from build123d import *

# Parameters (mm, degrees)
SKETCH1_R               = 13.5
BOSS_EXTRUDE1_DEPTH     = 1.75
CUT_EXTRUDE1_DEPTH      = 20.17191957
CIRPATTERN1_COUNT       = 4
CUT_EXTRUDE2_DEPTH      = 20.17191957
CUT_EXTRUDE2_DEPTH_BACK = 20.17191957
SKETCH3_W               = 4.596194078
SKETCH3_H               = 4.596194078
CHAMFER1_SIZE           = 0.5
SKETCH4_R               = 13.5
SKETCH4_R_2             = 12.5
CUT_EXTRUDE3_DEPTH      = 1


with BuildPart() as part:
    # Sketch1 → Boss-Extrude1 (new, symmetric)
    with BuildSketch(Plane(origin=(0, 0, 0), x_dir=(0, 0, -1), z_dir=(1, 0, 0))):
        Circle(SKETCH1_R)
    extrude(amount=BOSS_EXTRUDE1_DEPTH, both=True)

    # Sketch2 → Cut-Extrude1 (cut, symmetric)
    with BuildSketch(Plane(origin=(0, 0, 0), x_dir=(0, 0, -1), z_dir=(1, 0, 0))):
        with BuildLine():
            ThreePointArc((0, 3.587478321), (-3.402339743, 6.089548883), (-5.012219469, 9.99397715))
            ThreePointArc((-5.012219469, 9.99397715), (-2.621563936, 11.159720287), (0, 11.6087119))
            ThreePointArc((0, 11.6087119), (2.621563936, 11.159720287), (5.012219469, 9.99397715))
            ThreePointArc((5.012219469, 9.99397715), (3.402339743, 6.089548883), (0, 3.587478321))
        make_face()
    cut_extrude1 = extrude(amount=CUT_EXTRUDE1_DEPTH, both=True, mode=Mode.SUBTRACT)

    # CirPattern1: Cut-Extrude1 ×4 about axis
    cirpattern1_axis = Axis((0, 0, 0), (1, 0, 0))
    for i in range(1, CIRPATTERN1_COUNT):
        add(cut_extrude1.rotate(cirpattern1_axis, i * 360 / CIRPATTERN1_COUNT), mode=Mode.SUBTRACT)

    # Sketch3 → Cut-Extrude2 (cut, two sides: drawn at the far end of the back side and taken through both)
    with BuildSketch(Plane(origin=(0, 0, 0), x_dir=(0, 0, -1), z_dir=(1, 0, 0)).offset(-CUT_EXTRUDE2_DEPTH_BACK)):
        Rectangle(SKETCH3_W, SKETCH3_H)
    extrude(amount=CUT_EXTRUDE2_DEPTH + CUT_EXTRUDE2_DEPTH_BACK, mode=Mode.SUBTRACT)

    # Chamfer1
    chamfer1_edges = [part.edges().sort_by_distance(p)[0] for p in [
        (1.75, 0, 13.5),
        (1.75, 0, 2.298097039),
        (1.75, -2.298097039, 0),
        (1.75, 0, -2.298097039),
        (1.75, 2.298097039, 0),
    ]]
    chamfer(chamfer1_edges, length=CHAMFER1_SIZE)

    # Sketch4 → Cut-Extrude3 (cut, symmetric)
    with BuildSketch(Plane(origin=(0, 0, 0), x_dir=(0, 0, -1), z_dir=(1, 0, 0))):
        Circle(SKETCH4_R)
        Circle(SKETCH4_R_2, mode=Mode.SUBTRACT)
    extrude(amount=CUT_EXTRUDE3_DEPTH, both=True, mode=Mode.SUBTRACT)


solid = part.part
Check sheet for the modelled part. Datum: model origin and axes. Units: mm. A direction names the side the tool comes from. Give positions to 0.01 mm unless a question says otherwise; leave off trailing zeros. Order: outer loops, then holes, each group sorted by start corner. A loop starts at its lowest first (then second) coordinate and runs counter-clockwise, first axis right, second up. Notation, with made-up numbers: (33, 40.25) - (37, 40.25) arc R21 cw to (37, 49.25) - close; hole circle Ø7 at (77, 61.25). An arc over 180 degrees is marked (long way). Answer as CSV lines item,"result".
1. Section check B-B (z = -1.25). State how many separate pieces and enclosed holes the cut face has, then the cut area to 3 significant figures.
Result sheet:
separate pieces,"4"
enclosed holes,"0"
area,"22.4 mm²"
2. Section check A-A (x = -0.45). Record the boundary of the cut face in (y, z), then the cut area to 3 significant figures.
Result sheet:
outline,"circle Ø25 at (0, 0); hole (-11.61, 0) arc R9.39 ccw to (-9.99, -5.01) arc R7.84 ccw to (-3.59, 0) arc R7.84 ccw to (-9.99, 5.01) arc R9.39 ccw to start; hole (-5.01, -9.99) arc R9.39 ccw to (0, -11.61) arc R9.39 ccw to (5.01, -9.99) arc R7.84 ccw to (0, -3.59) arc R7.84 ccw to start; hole (-5.01, 9.99) arc R7.84 ccw to (0, 3.59) arc R7.84 ccw to (5.01, 9.99) arc R9.39 ccw to (0, 11.61) arc R9.39 ccw to start; hole (-2.3, -2.3) - (2.3, -2.3) - (2.3, 2.3) - (-2.3, 2.3) - close; hole (3.59, 0) arc R7.84 ccw to (9.99, -5.01) arc R9.39 ccw to (11.61, 0) arc R9.39 ccw to (9.99, 5.01) arc R7.84 ccw to start"
area,"248 mm²"
3. Mould release check, pull along Y, two halves, no side actions. Record for faces 1 (the face through (-1.37, -13.18, 2.93)), 2 (the face through (1.75, 3, 0)), 3 (the face through (0.02, -2.59, -11.17)): released by +Y, released by -Y, zero draft, split by the parting line, or undercut.
Result sheet:
face 1,"split by the parting line"
face 2,"zero draft"
face 3,"undercut"
4. Tool access check on faces 4 (the face through (-1.75, 0, -3)), 5 (the face through (-1, -9, -9)), 6 (the face through (0.024, -2.657, 11.148)). Record the directions out of +Z, -Z, +X, -X, +Y, -Y that give a thin tool (end or side, any length) a straight path to the whole face; none if there is none.
Result sheet:
face 4,"+Z, -Z, -X, +Y, -Y"
face 5,"none"
face 6,"+X, -X"
5. Go/stop test with flat-tipped pins: P1, Ø0.9, axis at x = 0, z = -1, coming from the +Y side; P2, Ø0.9, axis at x = 0, y = 0, coming from the -Z side; P3, Ø2, axis at x = 0.5, y = -2, coming from the -Z side. Record where each tip stops, or that it passes through.
Result sheet:
P1,"y = 12.49"
P2,"z = -12.5"
P3,"z = -13.45"
6. Scan lines: probe 1 along Y at (x, z) = (0.55, 2.5); probe 2 along Y at (x, z) = (0.7, 1.5); probe 3 along Y at (x, z) = (-1.15, 0.25). Record each from-to range of solid material in increasing order. Write a range as from..to.
Result sheet:
probe 1,"-12.25..-11.2, -5.12..5.12, 11.2..12.25"
probe 2,"-12.41..-11.45, -4.35..-2.3, 2.3..4.35, 11.45..12.41"
probe 3,"-13.5..-11.6, -3.69..-2.3, 2.3..3.69, 11.6..13.5"
